For this review, take the finished solid that the model builds, in its own axes (mm). Face numbers are marked on the shaded views. A direction names the side the tool comes from. Round coordinates to 2 decimals unless told otherwise and drop trailing zeros. Write each loop counter-clockwise with the first axis right and the second up, starting at its lowest first coordinate (ties: lowest second). Pieces come first, ordered by that corner, then holes. Notation, with made-up numbers: M 22,4 L 54,4 A4 cw 54,9 Z; hole C -16,-35.5 d1. An arc over 180 degrees is marked long. Answer in a Markdown table with one row per item.
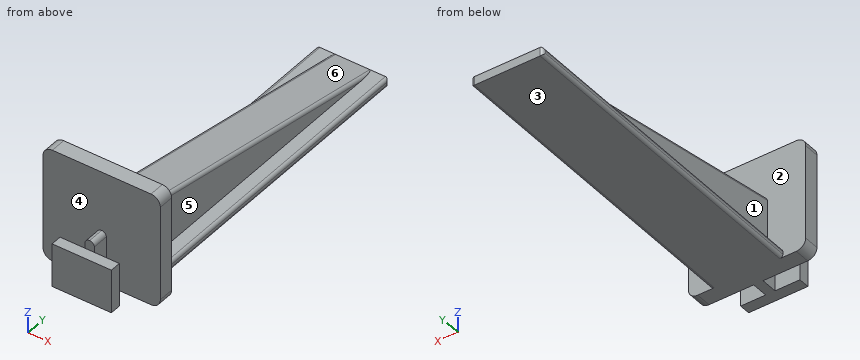
```python
from build123d import *

# Parameters (mm, degrees)
F0_W      = 37.62
F0_H      = 36.35
F1_DEPTH  = 5
F2_W      = 3
F2_H      = 17.2
F3_DEPTH  = 5.3
F4_W      = 19
F4_H      = 14
F5_DEPTH  = 3.5
F6_W      = 23
F6_H      = 22
F7_DEPTH  = 106
F9_DEPTH  = 25
F11_DEPTH = 5
F13_DEPTH = 5
F14_R     = 3
F16_DEPTH = 5.3
F17_R     = 1


with BuildPart() as f1:
    # F0 (on Front) → F1 (new body)
    with BuildSketch(Plane.XZ):
        with Locations((18.81, 18.175)):
            Rectangle(F0_W, F0_H)
    extrude(amount=F1_DEPTH)

    # F2 (on face) → F3 (join)
    with BuildSketch(Plane.XZ.offset(5)):
        with Locations((18.81, 8.6)):
            Rectangle(F2_W, F2_H)
    extrude(amount=F3_DEPTH)

    # F4 (on face) → F5 (join)
    with BuildSketch(Plane.XZ.offset(10.3)):
        with Locations((18.81, 7)):
            Rectangle(F4_W, F4_H)
    extrude(amount=F5_DEPTH)

    # F6 (on face) → F7 (join)
    with BuildSketch(Plane(origin=(0, 0, 0), x_dir=(-1, 0, 0), z_dir=(0, 1, 0))):
        with Locations((-18.81, 11)):
            Rectangle(F6_W, F6_H)
    extrude(amount=F7_DEPTH)

    # F8 (on face) → F9 (cut)
    with BuildSketch(Plane.YZ.offset(30.31)):
        Polygon((106, 22), (0, 22), (106, 2.8), align=None)
    extrude(amount=-F9_DEPTH, mode=Mode.SUBTRACT)

    # F10 (on face) → F11 (cut)
    with BuildSketch(Plane.YZ.offset(30.31)):
        Polygon((0, 2.8), (106, 2.8), (0, 22), align=None)
    extrude(amount=-F11_DEPTH, mode=Mode.SUBTRACT)

    # F12 (on face) → F13 (cut)
    with BuildSketch(Plane(origin=(7.31, 0, 0), x_dir=(0, -1, 0), z_dir=(-1, 0, 0))):
        Polygon((0, 22), (-106, 2.8), (0, 2.8), align=None)
    extrude(amount=-F13_DEPTH, mode=Mode.SUBTRACT)

    # F14
    f14_edges = [f1.edges().sort_by_distance(p)[0] for p in [
        (37.62, -2.5, 0),
        (37.62, -2.5, 36.35),
        (0, -2.5, 36.35),
        (0, -2.5, 0),
    ]]
    fillet(f14_edges, radius=F14_R)

    # F15 (on face) → F16 (cut, through all)
    with BuildSketch(Plane.XZ.offset(10.3)):
        with BuildLine():
            ThreePointArc((17.31, 15.79375), (17.7819509907, 16.79346061), (18.81, 17.2))
            Line((18.81, 17.2), (17.31, 17.2))
            Line((17.31, 17.2), (17.31, 15.79375))
        make_face()
        with BuildLine():
            ThreePointArc((18.81, 17.2), (19.8380490093, 16.79346061), (20.31, 15.79375))
            Line((20.31, 15.79375), (20.31, 17.2))
            Line((20.31, 17.2), (18.81, 17.2))
        make_face()
    extrude(amount=-F16_DEPTH, mode=Mode.SUBTRACT)

    # F17
    f17_edges = [f1.edges().sort_by_distance(p)[0] for p in [
        (30.31, 106, 1.4),
        (7.31, 106, 1.4),
        (7.31, 53, 2.8),
        (7.31, 53, 0),
        (25.31, 53, 12.4),
        (30.31, 53, 2.8),
        (30.31, 53, 0),
        (12.31, 53, 12.4),
    ]]
    fillet(f17_edges, radius=F17_R)


solid = f1.part
```
Q1. Take a section at A-A (x = 15). State the section outline as (y, z) points.
Found:
| item | result |
|---|---|
| outline | M -13.8,0 L -10.3,0 L -10.3,14 L -13.8,14 Z; M -5,0 L 106,0 L 106,2.8 L 0,22 L 0,36.35 L -5,36.35 Z |
Q2. Take a section at C-C (x = 33.5). State the section outline as (y, z) points, then the cut area to 3 significant figures.
Found:
| item | result |
|---|---|
| outline | M -5,0 L 0,0 L 0,36.35 L -5,36.35 Z |
| area | 182 mm² |
Q3. Machinability: for the marked faces 1, 2 and 3, which of the approach directions +Z, -Z, +X, -X, +Y, -Y give a long, thin tool a straight path to every point of the face, cutting with its end or side? Answer none if there is none.
Found:
| item | result |
|---|---|
| face 1 | +Z, -X, +Y |
| face 2 | +Z, +Y |
| face 3 | -Z, +X, -X, +Y, -Y |
Q4. Take a section at B-B (z = 30.5). State the section outline as (x, y) points.
Found:
| item | result |
|---|---|
| outline | M 0,-5 L 37.62,-5 L 37.62,0 L 0,0 Z |
Q5. For probe 1 along Y at (x, z) = (26.5, 3); probe 2 along X at (y, z) = (59, 6); probe 3 along Y at (x, z) = (20.5, 31), list the stretches that pass through material, from the lowest coordinate up.
Found:
| item | result |
|---|---|
| probe 1 | -13.8 to -10.3, -5 to 0 |
| probe 2 | 12.31 to 25.31 |
| probe 3 | -5 to 0 |
Q6. Mouldability with a two-part tool opening along Y and no side actions: class the marked faces 4, 5 and 6 as +Y half, -Y half, draft (parallel to the pull), parting line (faces both ways), or undercut.
Found:
| item | result |
|---|---|
| face 4 | undercut |
| face 5 | draft |
| face 6 | +Y half |
Q7. Insertion check: P1, Ø1.5, axis at x = 18.5, z = 15, coming from the -Y side; P2, Ø4, axis at x = 10, y = 67, coming from the +Z side; P3, Ø4, axis at x = 30.5, z = 8.5, coming from the -Y side. Each pin has a flat end and moves straight along its axis. Give the tip position at first contact, or say it passes through.
Found:
| item | result |
|---|---|
| P1 | y = -10.3 |
| P2 | z = 2.8 |
| P3 | y = -5 |
